```python
from build123d import *

# Parameters (mm, degrees)
CYLINDER003_R          = 5.85
CYLINDER003_DEPTH      = 30
CYLINDER002_R          = 9
CYLINDER002_DEPTH      = 30
CYLINDER001_R          = 7.35
CYLINDER001_DEPTH      = 25
LINEAREXTRUDE_DEPTH    = 12
CYLINDER_R             = 10.5
CYLINDER_DEPTH         = 25
DIFFERENCE_PITCH_ANGLE = 90


with BuildPart() as cylinder003:
    # cylinder003 → cylinder003 (new body)
    with BuildSketch(Plane.XY.offset(-5)):
        Circle(CYLINDER003_R)
    extrude(amount=CYLINDER003_DEPTH)


with BuildPart() as group001:
    # cylinder002 → cylinder002 (new body)
    with BuildSketch(Plane.XY.offset(-25)):
        Circle(CYLINDER002_R)
    extrude(amount=CYLINDER002_DEPTH)

    # Group001: union cylinder003
    add(cylinder003.part)


with BuildPart() as cylinder001:
    # cylinder001 → cylinder001 (new body)
    with BuildSketch(Plane.XY.offset(-2.5)):
        Circle(CYLINDER001_R)
    extrude(amount=CYLINDER001_DEPTH)


with BuildPart() as linearextrude:
    # RefineLinearExtrude → LinearExtrude (new body)
    with BuildSketch(Plane(origin=(0, 0, 0), x_dir=(0, -1, 0), z_dir=(0, 0, -1))):
        Polygon((-10.608811, -6.125), (0, -12.25), (10.608811, -6.125), (10.608811, 6.125), (0, 12.25), (-10.608811, 6.125), align=None)
    extrude(amount=-LINEAREXTRUDE_DEPTH)


with BuildPart() as linearextrude_1:
    # LinearExtrude placement: moved
    add(linearextrude.part.moved(Location((0, 0, -6))))


with BuildPart() as difference:
    # cylinder → cylinder (new body)
    with BuildSketch(Plane.XY.offset(-22.5)):
        Circle(CYLINDER_R)
    extrude(amount=CYLINDER_DEPTH)

    # Group: union cylinder001, LinearExtrude
    add(cylinder001.part)
    add(linearextrude_1.part)

    # difference: cut Group001
    add(group001.part, mode=Mode.SUBTRACT)


with BuildPart() as difference_1:
    # difference pitch: moved
    add(difference.part.rotate(Axis((0, 0, 0), (0, 1, 0)), DIFFERENCE_PITCH_ANGLE))


with BuildPart() as difference_2:
    # difference placement: moved
    add(difference_1.part)


solid = difference_2.part
```
Work out the finished part from the listing and answer in its coordinate system (mm). A direction names the side the tool comes from. Round coordinates to 2 decimals unless told otherwise and drop trailing zeros. Write each loop counter-clockwise with the first axis right and the second up, starting at its lowest first coordinate (ties: lowest second). Pieces come first, ordered by that corner, then holes.
1) Determine the mould class of faces 4 (the face through (0, -10.609, 0)), 5 (the face through (-14.4, 3.2, -10)), 6 (the face through (5, -6, 0)) for opening direction Z: pulls with the +Z half, pulls with the -Z half, needs draft (parallel to the pull), parting line crosses it, or undercut.
2) A cutting plane is placed at A-A on z = -4.5. Determine the outline of the cut face in (x, y), and give its area (3 significant figures).
3) A cutting plane is placed at D-D on z = 9.75. Determine the outline of the cut face in (x, y).
4) A cutting plane is placed at C-C on x = -4.5. Determine the outline of the cut face in (y, z) (3 decimals), and give its area (3 significant figures).
5) Consider probe 1 along Y at (x, z) = (-3.5, 0); probe 2 along Z at (x, y) = (-13, 0); probe 3 along Z at (x, y) = (-0.5, 0). Determine where each line is inside the solid, lowest interval first.
6) Which of the six approach directions +Z, -Z, +X, -X, +Y, -Y give full straight-line access (tool end or side, diameter ignored) to faces 1 (the face through (6, 7, -3)), 2 (the face through (-0.084, 5.379, -9.145)), 3 (the face through (-8.943, 8.923, 1.172))?
7) A cutting plane is placed at B-B on y = -4.75. Determine the outline of the cut face in (x, z), and give its area (3 significant figures).
8) Flat-ended cylindrical pins translate along their axes: P1, Ø12, axis at x = 16.5, z = -7, coming from the +Y side; P2, Ø10, axis at x = -17, z = 5, coming from the -Y side; P3, Ø6, axis at x = -3.5, y = 4, coming from the -Z side. Find the tip coordinate at first contact, or state that the pin passes through.
Entries:
1. face 4: needs draft
1. face 5: parting line crosses it
1. face 6: undercut
2. outline: (-22.5, -9.49) - (-6, -9.49) - (-6, -10.61) - (6, -10.61) - (6, -5.81) - (22.5, -5.81) - (22.5, -3.74) - (5, -3.74) - (5, -7.79) - (-22.5, -7.79) - close; (-22.5, 7.79) - (5, 7.79) - (5, 3.74) - (22.5, 3.74) - (22.5, 5.81) - (6, 5.81) - (6, 10.61) - (-6, 10.61) - (-6, 9.49) - (-22.5, 9.49) - close
2. area: 200 mm2
3. outline: (-22.5, -3.9) - (-6, -3.9) - (-6, -4.33) - (6, -4.33) - (6, 4.33) - (-6, 4.33) - (-6, 3.9) - (-22.5, 3.9) - close
4. outline: (-10.609, -6.125) - (0, -12.25) - (10.609, -6.125) - (10.609, 6.125) - (0, 12.25) - (-10.609, 6.125) - close; hole circle Ø18 at (0, 0)
4. area: 135 mm2
5. probe 1: y = -10.61 to -9, 9 to 10.61
5. probe 2: z = -10.5 to -9, 9 to 10.5
5. probe 3: z = -12.25 to -9, 9 to 12.25
6. face 1: +X
6. face 2: -Z, +X, -X, +Y
6. face 3: -X
7. outline: (-22.5, -9.36) - (-6, -9.36) - (-6, -9.51) - (6, -9.51) - (6, -5.61) - (22.5, -5.61) - (22.5, -3.41) - (5, -3.41) - (5, -7.64) - (-22.5, -7.64) - close; (-22.5, 7.64) - (5, 7.64) - (5, 3.41) - (22.5, 3.41) - (22.5, 5.61) - (6, 5.61) - (6, 9.51) - (-6, 9.51) - (-6, 9.36) - (-22.5, 9.36) - close
7. area: 182 mm2
8. P1: stops at y = 7.28
8. P2: stops at y = -10.5
8. P3: stops at z = -11.67
